Could you check a few things on this model? Use its own coordinates, in mm. A direction names the side the tool comes from. Give positions to 0.01 mm unless a question says otherwise; leave off trailing zeros. Write each loop counter-clockwise with the first axis right and the second up, starting at its lowest first coordinate (ties: lowest second). Pieces come first, ordered by that corner, then holes. Notation, with made-up numbers: M 49.25,60 L 103.25,60 A22 cw 103.25,94 Z; hole C 17.5,-31 d7. An arc over 180 degrees is marked long. One line per item, written item: value.
```python
from build123d import *

# Parameters (mm, degrees)
SKETCH_1_R      = 5
SKETCH_1_R_2    = 1.6
EXTRUDE_1_DEPTH = 40


with BuildPart() as part:
    # 草图1 → 凸台-拉伸1 (new body)
    with BuildSketch(Plane(origin=(0, 0, 0), x_dir=(1, 0, 0), z_dir=(0, 1, 0))):
        with Locations(Location((0, 0, 0), (0, 0, 270))):
            Circle(SKETCH_1_R)
        with Locations(Location((0, 0, 0), (0, 0, 270))):
            Circle(SKETCH_1_R_2, mode=Mode.SUBTRACT)
        with BuildLine():
            ThreePointArc((4.285732143, 0.35), (3.040559159, 3.040559159), (0.35, 4.285732143))
            Line((0.35, 4.285732143), (0.35, 2.576334606))
            ThreePointArc((0.35, 2.576334606), (1.838477631, 1.838477631), (2.576334606, 0.35))
            Line((2.576334606, 0.35), (4.285732143, 0.35))
        make_face(mode=Mode.SUBTRACT)
        with BuildLine():
            ThreePointArc((0.35, -4.285732143), (3.040559159, -3.040559159), (4.285732143, -0.35))
            Line((4.285732143, -0.35), (2.576334606, -0.35))
            ThreePointArc((2.576334606, -0.35), (1.838477631, -1.838477631), (0.35, -2.576334606))
            Line((0.35, -2.576334606), (0.35, -4.285732143))
        make_face(mode=Mode.SUBTRACT)
        with BuildLine():
            ThreePointArc((-4.285732143, -0.35), (-3.040559159, -3.040559159), (-0.35, -4.285732143))
            Line((-0.35, -4.285732143), (-0.35, -2.576334606))
            ThreePointArc((-0.35, -2.576334606), (-1.838477631, -1.838477631), (-2.576334606, -0.35))
            Line((-2.576334606, -0.35), (-4.285732143, -0.35))
        make_face(mode=Mode.SUBTRACT)
        with BuildLine():
            ThreePointArc((-0.35, 4.285732143), (-3.040559159, 3.040559159), (-4.285732143, 0.35))
            Line((-4.285732143, 0.35), (-2.576334606, 0.35))
            ThreePointArc((-2.576334606, 0.35), (-1.838477631, 1.838477631), (-0.35, 2.576334606))
            Line((-0.35, 2.576334606), (-0.35, 4.285732143))
        make_face(mode=Mode.SUBTRACT)
    extrude(amount=EXTRUDE_1_DEPTH)


solid = part.part
```
1) I'm going to push flat-ended pins straight in: pin 1 (5 mm diameter, centred on x = 4, y = 9.5, fed in from +Z); pin 2 (0.5 mm diameter, centred on y = 10, z = -3, fed in from +X); pin 3 (0.9 mm diameter, centred on x = -3.5, y = 28, fed in from -Z). Where does each tip first touch, or does it pass through?
Outcome:
pin 1: stops at z = 4.77
pin 2: stops at x = 4.18
pin 3: stops at z = -3.96
2) If we section it at A-A, the plane x = 0: Write out the boundary of the cut face in (y, z).
Outcome:
outline: M 0,-5 L 40,-5 L 40,-1.6 L 0,-1.6 Z; M 0,1.6 L 40,1.6 L 40,5 L 0,5 Z
3) If we section it at D-D, the plane z = 2: Write out the boundary of the cut face in (x, y), then the cut area to 3 significant figures.
Outcome:
outline: M -4.58,0 L -3.81,0 L -3.81,40 L -4.58,40 Z; M -1.66,0 L 1.66,0 L 1.66,40 L -1.66,40 Z; M 3.81,0 L 4.58,0 L 4.58,40 L 3.81,40 Z
area: 195 mm^2
4) If we section it at C-C, the plane y = 22.5: Write out the boundary of the cut face in (x, z), then the cut area to 3 significant figures.
Outcome:
outline: C 0,0 d10; hole M -4.29,-0.35 A4.3 ccw -0.35,-4.29 L -0.35,-2.58 A2.6 cw -2.58,-0.35 Z; hole M -4.29,0.35 L -2.58,0.35 A2.6 cw -0.35,2.58 L -0.35,4.29 A4.3 ccw Z; hole C 0,0 d3.2; hole M 0.35,-4.29 A4.3 ccw 4.29,-0.35 L 2.58,-0.35 A2.6 cw 0.35,-2.58 Z; hole M 0.35,2.58 A2.6 cw 2.58,0.35 L 4.29,0.35 A4.3 ccw 0.35,4.29 Z
area: 38.4 mm^2
5) Please list where these lines run through material, in increasing order: L1, parallel to X at y = 17.5, z = 0; L2, parallel to Z at x = -0.5, y = 18; L3, parallel to X at y = 20, z = 1.75. Write a range as from..to.
Outcome:
L1: x = -5..-1.6, 1.6..5
L2: z = -4.97..-4.27, -2.55..-1.52, 1.52..2.55, 4.27..4.97
L3: x = -4.68..-3.93, -1.92..1.92, 3.93..4.68
6) We'd pull the mould along X, two halves only. Please class faces 1 (the face through (0, 0, 2)), 2 (the face through (-3.07, 19.72, 3.01)), 3 (the face through (-4.88, 19.72, -1.08)): pulls with the +X half, pulls with the -X half, needs draft (parallel to the pull), parting line crosses it, or undercut.
Outcome:
face 1: needs draft
face 2: undercut
face 3: parting line crosses it
7) On a 3-axis mill with a long thin cutter (end or side, diameter ignored), from which of +Z, -Z, +X, -X, +Y, -Y can I reach the whole of each face in a straight line? I mean faces 4 (the face through (3, 20, -0.35)), 5 (the face through (0, 40, 2)). Say none if no direction works.
Outcome:
face 4: +Y, -Y
face 5: +Z, -Z, +X, -X, +Y
8) If we section it at B-B, the plane z = 0: Write out the boundary of the cut face in (x, y).
Outcome:
outline: M -5,0 L -1.6,0 L -1.6,40 L -5,40 Z; M 1.6,0 L 5,0 L 5,40 L 1.6,40 Z
